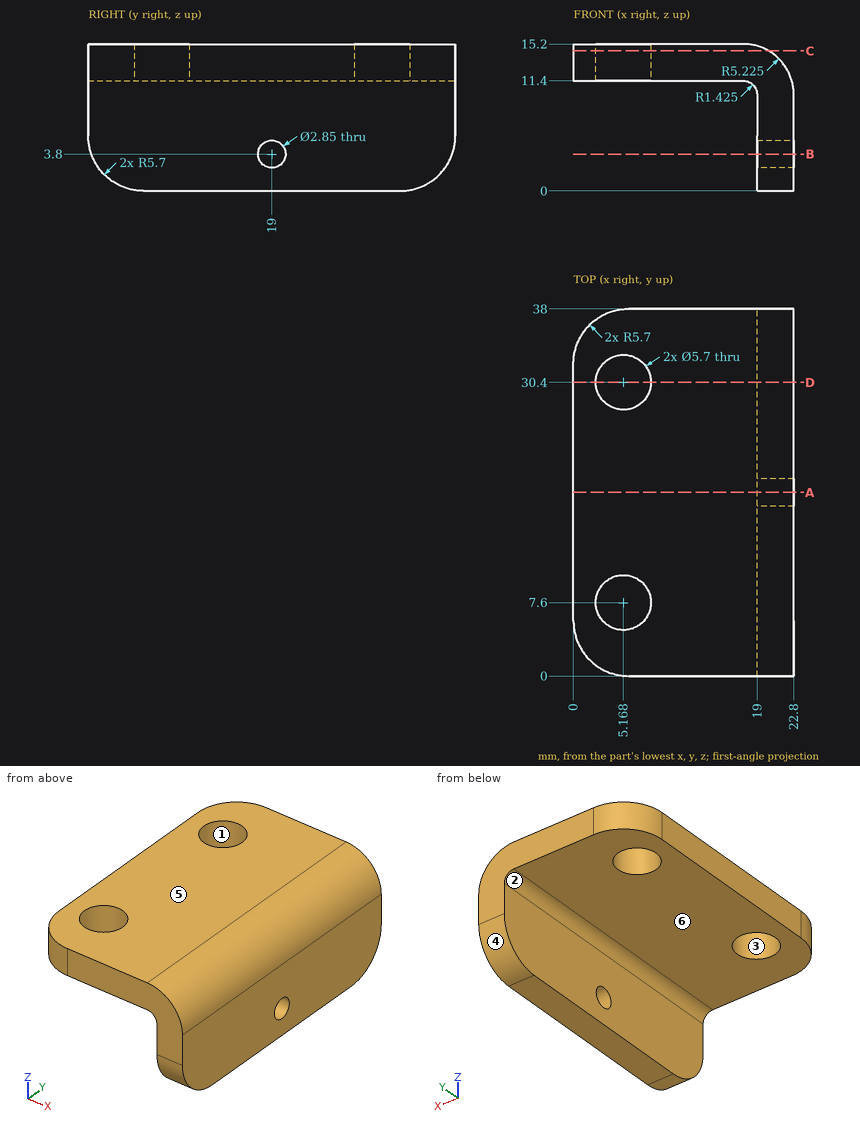
Here's the drawing with two shaded views (mm, measured from the low corner). I have some questions. A direction names the side the tool comes from. Give positions to 0.01 mm unless a question says otherwise; leave off trailing zeros. Loops run counter-clockwise (first coordinate to the right, second up) from the corner with the lowest first, then second, coordinate; pieces in that order, holes last. Notation, with made-up numbers: M 65,87.25 L 110,87.25 A16 cw 110,116.25 Z; hole C 7,57 d8. An arc over 180 degrees is marked long. Answer in a Markdown table with one row per item.
1. Suppose I cut it at B-B on z = 3.8. Write out the boundary of the cut face in (x, y) (3 decimals).
Taken from the geometry:
| item | result |
|---|---|
| outline | M 19,0.326 L 22.8,0.326 L 22.8,17.575 L 19,17.575 Z; M 19,20.425 L 22.8,20.425 L 22.8,37.674 L 19,37.674 Z |
2. For pin 1 Ø1.5 at (x, y) = (14, 27) entering from -Z, with a flat end and sliding along its axis, tell me the tip position at first contact or that it passes through.
Taken from the geometry:
| item | result |
|---|---|
| pin 1 | stops at z = 11.4 |
3. Suppose I cut it at D-D on y = 30.4. Write out the boundary of the cut face in (x, z) (3 decimals), plus the area to 3 significant figures.
Taken from the geometry:
| item | result |
|---|---|
| outline | M 0,11.4 L 2.318,11.4 L 2.318,15.2 L 0,15.2 Z; M 8.018,11.4 L 17.575,11.4 A1.425 cw 19,9.975 L 19,0 L 22.8,0 L 22.8,9.975 A5.225 ccw 17.575,15.2 L 8.018,15.2 Z |
| area | 103 mm² |
4. If I drill on line 1 along Z through (x, y) = (4.75, 14); line 2 along Y through (x, z) = (6.5, 12.75); line 3 along Y through (x, z) = (20.85, 3.8) (3 decimals), over which ranges is the centre line in solid material (lowest first)?
Taken from the geometry:
| item | result |
|---|---|
| line 1 | z = 11.4 to 15.2 |
| line 2 | y = 0 to 5.08, 10.12 to 27.88, 32.92 to 38 |
| line 3 | y = 0.326 to 17.575, 20.425 to 37.674 |
5. Which directions (+Z, -Z, +X, -X, +Y, -Y) give clear straight access to the entire face, cutting with the end or side of a thin tool? Please do the marked faces 5 and 6.
Taken from the geometry:
| item | result |
|---|---|
| face 5 | +Z, +X, -X, +Y, -Y |
| face 6 | -Z, -X, +Y, -Y |
6. Thinking about a two-plate mould opening in X: for the marked faces 1, 2, 3 and 4, which applies, released by +X, released by -X, zero draft, split by the parting line, or undercut?
Taken from the geometry:
| item | result |
|---|---|
| face 1 | undercut |
| face 2 | released by -X |
| face 3 | undercut |
| face 4 | zero draft |
7. Suppose I cut it at C-C on z = 14.5. Write out the boundary of the cut face in (x, y), plus the area to 3 significant figures.
Taken from the geometry:
| item | result |
|---|---|
| outline | M 0,5.7 A5.7 ccw 5.7,0 L 20.19,0 L 20.19,38 L 5.7,38 A5.7 ccw 0,32.3 Z; hole C 5.17,7.6 d5.7; hole C 5.17,30.4 d5.7 |
| area | 702 mm² |
8. Suppose I cut it at A-A on y = 19. Write out the boundary of the cut face in (x, z) (3 decimals), plus the area to 3 significant figures.
Taken from the geometry:
| item | result |
|---|---|
| outline | M 0,11.4 L 17.575,11.4 A1.425 cw 19,9.975 L 19,5.225 L 22.8,5.225 L 22.8,9.975 A5.225 ccw 17.575,15.2 L 0,15.2 Z; M 19,0 L 22.8,0 L 22.8,2.375 L 19,2.375 Z |
| area | 114 mm² |
